Input: part model. Units: mm. Frame: model coordinates. A direction names the side the tool comes from. Round coordinates to 2 decimals unless told otherwise and drop trailing zeros. Order: outer loops, then holes, each group sorted by start corner. A loop starts at its lowest first (then second) coordinate and runs counter-clockwise, first axis right, second up. Notation, with made-up numbers: (1, 48.25) -> (44, 48.25) arc R4 ccw to (44, 55.25) -> close; hole circle Ø8 at (-34, -21.75). An arc over 180 degrees is marked (long way). Use a Markdown table: item, result.
from build123d import *

# Parameters (mm, degrees)
F0_W     = 57.15
F0_H     = 31.75
F1_DEPTH = 38.1
F3_DEPTH = 12.7
F5_DEPTH = 12.7
F7_DEPTH = 12.7


with BuildPart() as f1:
    # F0 (on Front) → F1 (new body)
    with BuildSketch(Plane.XZ):
        with Locations((28.575, 15.875)):
            Rectangle(F0_W, F0_H)
    extrude(amount=F1_DEPTH)

    # F2 (on face) → F3 (cut)
    with BuildSketch(Plane.XZ.offset(38.1)):
        Polygon((57.15, 31.75), (19.05, 31.75), (31.75, 0), (57.15, 0), align=None)
    extrude(amount=-F3_DEPTH, mode=Mode.SUBTRACT)

    # F4 (on face) → F5 (cut)
    with BuildSketch(Plane.XZ.offset(25.4)):
        Polygon((57.15, 31.75), (50.8, 31.75), (57.15, 0), align=None)
    extrude(amount=-F5_DEPTH, mode=Mode.SUBTRACT)

    # F6 (on face) → F7 (cut)
    with BuildSketch(Plane(origin=(0, 0, 0), x_dir=(-1, 0, 0), z_dir=(0, 1, 0))):
        Polygon((-38.1, 0), (-19.05, 31.75), (-57.15, 31.75), (-57.15, 0), align=None)
    extrude(amount=-F7_DEPTH, mode=Mode.SUBTRACT)


solid = f1.part
1) Set-up query: faces 1 (the flat face through (28.71, -6.26, 15.65)), 2 (the flat face through (15, 0, 16)), 3 (the flat face through (38, -25.4, 16)). Return all of +Z, -Z, +X, -X, +Y, -Y with unobstructed straight access to the full face (end or side cutting, diameter ignored); none if empty.
Results found:
| item | result |
|---|---|
| face 1 | +Z, +X, +Y |
| face 2 | +Z, -Z, +X, -X, +Y |
| face 3 | +Z, +X, -Y |
2) Cut plane A-A on z = 18.5. Return loops of the section in (x, y), and give its area (3 significant figures).
Results found:
| item | result |
|---|---|
| outline | (0, -38.1) -> (24.35, -38.1) -> (24.35, -25.4) -> (53.45, -25.4) -> (53.45, -12.7) -> (27, -12.7) -> (27, 0) -> (0, 0) -> close |
| area | 1,330 mm² |
3) Cut plane C-C on y = -8. Return loops of the section in (x, z).
Results found:
| item | result |
|---|---|
| outline | (0, 0) -> (38.1, 0) -> (19.05, 31.75) -> (0, 31.75) -> close |
4) Cut plane D-D on x = 53. Return loops of the section in (y, z).
Results found:
| item | result |
|---|---|
| outline | (-25.4, 0) -> (-12.7, 0) -> (-12.7, 20.75) -> (-25.4, 20.75) -> close |
5) Pin query (flat end, axial travel): pin 1 Ø1.5 at (x, z) = (27, 19) entering from -Y; pin 2 Ø5 at (y, z) = (-32, 23) entering from +X; pin 3 Ø8 at (y, z) = (-23, 4.5) entering from +X. Return the tip coordinate at first contact, or that it passes through.
Results found:
| item | result |
|---|---|
| pin 1 | stops at y = -25.4 |
| pin 2 | stops at x = 23.55 |
| pin 3 | stops at x = 57.05 |
6) Line query: L1, parallel to Y at x = 51.5, z = 10; L2, parallel to X at y = -7, z = 22; L3, parallel to X at y = -7, z = 28.5. Output: solid intervals per line, ascending. Write a range as [from, to].
Results found:
| item | result |
|---|---|
| L1 | y = [-25.4, -12.7] |
| L2 | x = [0, 24.9] |
| L3 | x = [0, 21] |
7) Cut plane B-B on x = 21. Return loops of the section in (y, z) (3 decimals), and give its area (3 significant figures).
Results found:
| item | result |
|---|---|
| outline | (-38.1, 0) -> (0, 0) -> (0, 28.5) -> (-12.7, 28.5) -> (-12.7, 31.75) -> (-25.4, 31.75) -> (-25.4, 26.875) -> (-38.1, 26.875) -> close |
| area | 1,110 mm² |
